from build123d import *

# Parameters (mm, degrees)
F2_DEPTH = 2
F3_W     = 10
F3_H     = 224
F4_DEPTH = 2


with BuildPart() as f2:
    # F1 (on face) → F2 (new body)
    with BuildSketch(Plane.XY):
        Polygon((10, 300), (0, 300), (0, 224), (0, 0), (10, 0), align=None)
    extrude(amount=F2_DEPTH)

    # F3 (on face) → F4 (join)
    with BuildSketch(Plane.XY.offset(2)):
        with Locations((5, 112)):
            Rectangle(F3_W, F3_H)
    extrude(amount=F4_DEPTH)


solid = f2.part
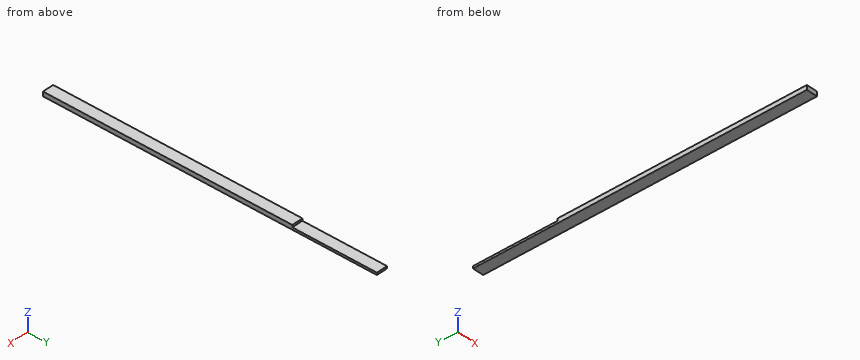
Here's how the part is built. I have some questions about the finished solid (model axes, mm). Round coordinates to 2 decimals unless told otherwise and drop trailing zeros. Loops run counter-clockwise (first coordinate to the right, second up) from the corner with the lowest first, then second, coordinate; pieces in that order, holes last.
1. If we section it at A-A on x = 1.5: Write out the boundary of the cut face in (y, z).
Answer list:
outline: (0, 0) - (300, 0) - (300, 2) - (224, 2) - (224, 4) - (0, 4) - close
2. For P1, Ø2, axis at x = 1.5, z = 1, coming from the -Y side; P2, Ø1, axis at x = 6, z = 3, coming from the +Y side, each with a flat end and sliding along its axis, tell me the tip position at first contact or that it passes through.
Answer list:
P1: stops at y = 0
P2: stops at y = 224
3. If we section it at C-C on y = 260: Write out the boundary of the cut face in (x, z), plus the area to 3 significant figures.
Answer list:
outline: (0, 0) - (10, 0) - (10, 2) - (0, 2) - close
area: 20.0 mm2
4. If I drill on line 1 along Y through (x, z) = (5.75, 2.45); line 2 along Z through (x, y) = (9, 238), over which ranges is the centre line in solid material (lowest first)?
Answer list:
line 1: y = 0 to 224
line 2: z = 0 to 2
5. If we section it at B-B on z = 3.15: Write out the boundary of the cut face in (x, y).
Answer list:
outline: (0, 0) - (10, 0) - (10, 224) - (0, 224) - close
